Work out the finished part from the listing and answer in its coordinate system (mm). A direction names the side the tool comes from. Coordinates: 2 decimals unless noted, no trailing zeros. Order: outer loops, then holes, each group sorted by start corner. A loop starts at its lowest first (then second) coordinate and runs counter-clockwise, first axis right, second up. Notation, with made-up numbers: M 34.5,61 L 39.5,61 A15 ccw 39.5,84 Z; hole C -20.75,-40 d5. An arc over 180 degrees is marked long. Write item = value, one per line. Start each with the question number.
Q1. Find section C-C on x = 25.5. Give the vertices of the cut face in (y, z).
Q2. A tool of negligible diameter and unlimited length cuts with its end or side. For faces 4 (the flat face through (2.1, 26.6, 16.7)), 5 (the flat face through (81, 10, 18)), from which of +Z, -Z, +X, -X, +Y, -Y can it reach the whole face along a straight path? Write none if from no direction.
Q3. Determine the mould class of faces 1 (the flat face through (78.9, 26.6, 16.7)), 2 (the flat face through (40, 14, 0)), 3 (the flat face through (57, 0, 18)) for opening direction Y: released by +Y, released by -Y, zero draft, split by the parting line, or undercut.
Q4. Straight lines are drawn through the part: line 1 along X through (y, z) = (3, 21); line 2 along Y through (x, z) = (26.5, 17.5); line 3 along X through (y, z) = (22, 25.5). For each, find the intervals that lie inside material, in ascending order.
Q5. Find section B-B on y = 27. Give the vertices of the cut face in (x, z).
Q6. Find section A-A on z = 10.5. Give the vertices of the cut face in (x, y), and give its area (3 significant figures).
Q7. Find section D-D on y = 3. Give the vertices of the cut face in (x, z), and give its area (3 significant figures).
```python
from build123d import *

# Parameters (mm, degrees)
SKETCH_1_W           = 81
SKETCH_1_H           = 28.5
EXTRUDE_1_DEPTH      = 3
EXTRUDE_2_DEPTH      = 30
EXTRUDE_2_DEPTH_BACK = 3
SKETCH_2_W           = 87
SKETCH_2_H           = 34.5
SKETCH_2_W_2         = 81
SKETCH_2_H_2         = 28.5
SKETCH_3_W           = 4
SKETCH_3_H           = 28.5
EXTRUDE_3_DEPTH      = 30
EXTRUDE_4_DEPTH      = 30
CHAMFER_1_SIZE       = 10


with BuildPart() as part:
    # 草图1 → 凸台-拉伸1 (new body)
    with BuildSketch(Plane.XY):
        with Locations((40.5, 14.25)):
            Rectangle(SKETCH_1_W, SKETCH_1_H)
    extrude(amount=EXTRUDE_1_DEPTH)

    # 草图2 → 凸台-拉伸2 (add, two sides: drawn at the far end of the back side and taken through both)
    with BuildSketch(Plane.XY.offset(3).offset(-EXTRUDE_2_DEPTH_BACK)):
        with Locations((40.5, 14.25)):
            Rectangle(SKETCH_2_W, SKETCH_2_H)
        with Locations((40.5, 14.25)):
            Rectangle(SKETCH_2_W_2, SKETCH_2_H_2, mode=Mode.SUBTRACT)
    extrude(amount=EXTRUDE_2_DEPTH + EXTRUDE_2_DEPTH_BACK)

    # 草图3 → 凸台-拉伸3 (add)
    with BuildSketch(Plane.XY.offset(3)):
        with Locations((32, 14.25)):
            Rectangle(SKETCH_3_W, SKETCH_3_H)
    extrude(amount=EXTRUDE_3_DEPTH)

    # 草图4 → 凸台-拉伸4 (add)
    with BuildSketch(Plane.XY.offset(3)):
        Polygon((-3, 16.5), (12, 31.5), (-3, 31.5), align=None)
        Polygon((69, 31.5), (84, 16.5), (84, 31.5), align=None)
    extrude(amount=EXTRUDE_4_DEPTH)

    # 倒角1
    chamfer_1_edges = [part.edges().sort_by_distance(p)[0] for p in [
        (-3, 31.5, 16.5),
        (84, 31.5, 16.5),
    ]]
    chamfer(chamfer_1_edges, length=CHAMFER_1_SIZE)


solid = part.part
```
Findings below:
q1.outline = M -3,0 L 31.5,0 L 31.5,33 L 28.5,33 L 28.5,3 L 0,3 L 0,33 L -3,33 Z
q2.face_4 = +Z, -Z, -X, +Y
q2.face_5 = +Z
q3.face_1 = released by +Y
q3.face_2 = zero draft
q3.face_3 = undercut
q4.line_1 = -3 to 0, 30 to 34, 81 to 84
q4.line_2 = -3 to 0, 28.5 to 31.5
q4.line_3 = -2.5 to 2.5, 30 to 34, 78.5 to 83.5
q5.outline = M 2.5,0 L 78.5,0 L 78.5,33 L 73.5,33 L 73.5,3 L 34,3 L 34,33 L 30,33 L 30,3 L 7.5,3 L 7.5,33 L 2.5,33 Z
q6.outline = M -3,-3 L 84,-3 L 84,21.5 L 74,31.5 L 7,31.5 L -3,21.5 Z; hole M 0,0 L 30,0 L 30,28.5 L 9,28.5 L 0,19.5 Z; hole M 34,0 L 81,0 L 81,19.5 L 72,28.5 L 34,28.5 Z
q6.area = 788 mm^2
q7.outline = M -3,0 L 84,0 L 84,33 L 81,33 L 81,3 L 34,3 L 34,33 L 30,33 L 30,3 L 0,3 L 0,33 L -3,33 Z
q7.area = 561 mm^2
